```python
from build123d import *

# Parameters (mm, degrees)
HOLE_WIZARD_M201_D           = 17.5
HOLE_WIZARD_M201_CSINK_D     = 20.05
HOLE_WIZARD_M201_CSINK_ANGLE = 90
SKETCH_4_R                   = 2.75
CUT_EXTRUDE_1_DEPTH          = 54.141321022


with BuildPart() as part:
    # Sketch 1 → Revolve 1 (revolve)
    with BuildSketch(Plane.XY, mode=Mode.PRIVATE) as revolve_1_sk:
        Polygon((0, 0), (-30, 0), (-30, 8), (-15, 8), (-15, 40), (0, 40), align=None)
    revolve(revolve_1_sk.sketch.rotate(Axis((0, 20.983482592, 0), (0, -1, 0)), 270), axis=Axis((0, 20.983482592, 0), (0, -1, 0)))

    # Hole Wizard M201 (through all)
    with Locations(Plane(origin=(0, 40, 0), x_dir=(1, 0, 0), z_dir=(0, 1, 0))):
        with Locations((0, 0)):
            CounterSinkHole(HOLE_WIZARD_M201_D / 2, HOLE_WIZARD_M201_CSINK_D / 2, counter_sink_angle=HOLE_WIZARD_M201_CSINK_ANGLE)

    # Sketch 4 → Cut-Extrude 1 (cut, through all)
    with BuildSketch(Plane(origin=(0, 8, 0), x_dir=(1, 0, 0), z_dir=(0, 1, 0))):
        with Locations(Location((-17.67766953, 17.67766953, 0), (0, 0, 270))):
            Circle(SKETCH_4_R)
        with Locations(Location((-17.67766953, -17.67766953, 0), (0, 0, 270))):
            Circle(SKETCH_4_R)
        with Locations(Location((17.67766953, 17.67766953, 0), (0, 0, 270))):
            Circle(SKETCH_4_R)
        with Locations(Location((17.67766953, -17.67766953, 0), (0, 0, 270))):
            Circle(SKETCH_4_R)
    extrude(amount=-CUT_EXTRUDE_1_DEPTH, mode=Mode.SUBTRACT)


solid = part.part
```
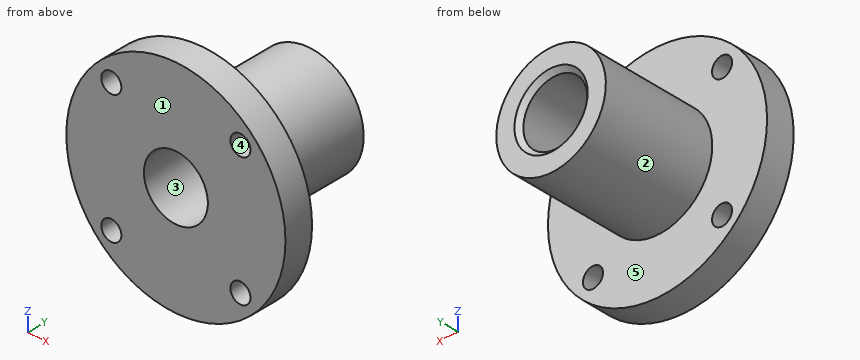
Here's how the part is built. I have some questions about the finished solid (model axes, mm). Face numbers are marked on the shaded views. A direction names the side the tool comes from. Coordinates: 2 decimals unless noted, no trailing zeros. Order: outer loops, then holes, each group sorted by start corner. A loop starts at its lowest first (then second) coordinate and runs counter-clockwise, first axis right, second up. Notation, with made-up numbers: M -24,57 L -15,57 A4 cw -15,62 Z; hole C 0,19.25 d2. An arc over 180 degrees is marked long. Answer as a JSON object with one key per item and string values. Group by question number.
(1) For pin 1 (14 mm diameter, centred on x = 0, z = 0, fed in from +Y); pin 2 (1.5 mm diameter, centred on y = 20.5, z = -14.5, fed in from -X); pin 3 (8 mm diameter, centred on y = 28.5, z = -7.5, fed in from +X); pin 4 (6 mm diameter, centred on x = -7, y = 8.5, fed in from +Z), each with a flat end and sliding along its axis, tell me the tip position at first contact or that it passes through.
(2) Suppose I cut it at A-A, the plane z = 0. Please give me the cut outline in (x, y) (3 decimals), then the cut area to 3 significant figures.
(3) If we mould it in two halves opening along X, with no side actions, what happens to the marked faces 1, 2 and 3? For each: released by +X, released by -X, zero draft, split by the parting line, or undercut.
(4) Which directions (+Z, -Z, +X, -X, +Y, -Y) give clear straight access to the entire face, cutting with the end or side of a thin tool? Please do the marked faces 4 and 5.
(5) Suppose I cut it at D-D, the plane y = 6.5. Please give me the cut outline in (x, z), then the cut area to 3 significant figures.
(6) Suppose I cut it at C-C, the plane y = 11. Please give me the cut outline in (x, z).
(7) Suppose I cut it at B-B, the plane x = 0. Please give me the cut outline in (y, z) (3 decimals).
(8) I need wall thicknesses on probe 1 along Z at (x, y) = (-16, 5); probe 2 along Y at (x, z) = (-14.5, -21); probe 3 along Z at (x, y) = (-0.5, 10.5). Which ranges of each line are inside material? Lowest first, please.
Values found:
{
 "1": {"pin 1": "passes through", "pin 2": "stops at x = -5.99", "pin 3": "stops at x = 14.59", "pin 4": "stops at z = 29.73"},
 "2": {"outline": "M -30,0 L -8.75,0 L -8.75,38.725 L -10.025,40 L -15,40 L -15,8 L -30,8 Z; M 8.75,0 L 30,0 L 30,8 L 15,8 L 15,40 L 10.025,40 L 8.75,38.725 Z", "area": "738 mm^2"},
 "3": {"face 1": "zero draft", "face 2": "split by the parting line", "face 3": "undercut"},
 "4": {"face 4": "+Y, -Y", "face 5": "+Y"},
 "5": {"outline": "C 0,0 d60; hole C -17.68,-17.68 d5.5; hole C -17.68,17.68 d5.5; hole C 0,0 d17.5; hole C 17.68,-17.68 d5.5; hole C 17.68,17.68 d5.5", "area": "2,490 mm^2"},
 "6": {"outline": "C 0,0 d30; hole C 0,0 d17.5"},
 "7": {"outline": "M 0,-30 L 8,-30 L 8,-15 L 40,-15 L 40,-10.025 L 38.725,-8.75 L 0,-8.75 Z; M 0,8.75 L 38.725,8.75 L 40,10.025 L 40,15 L 8,15 L 8,30 L 0,30 Z"},
 "8": {"probe 1": "z = -25.38 to -19.86, -15.5 to 15.5, 19.86 to 25.38", "probe 2": "y = 0 to 8", "probe 3": "z = -14.99 to -8.74, 8.74 to 14.99"}
}
